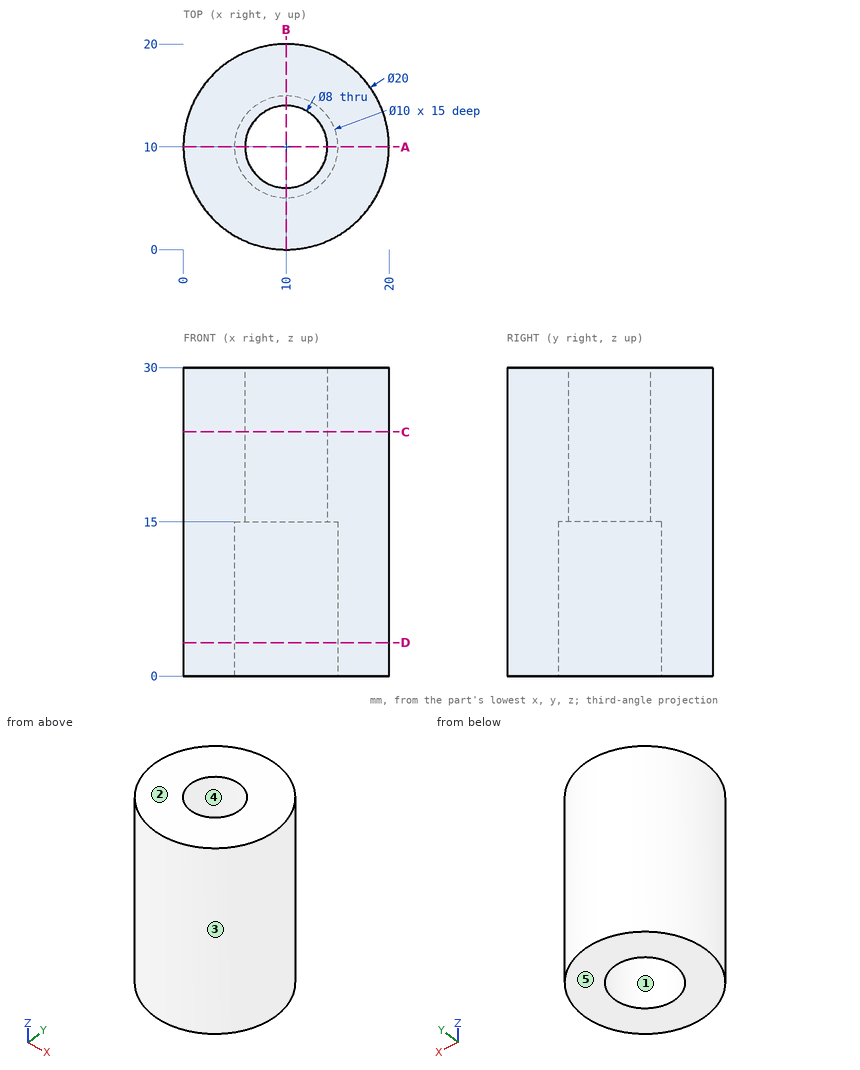
Can you work these out from the drawing? Everything is in mm from the part's minimum corner. A direction names the side the tool comes from. Round coordinates to 2 decimals unless told otherwise and drop trailing zeros. Loops run counter-clockwise (first coordinate to the right, second up) from the corner with the lowest first, then second, coordinate; pieces in that order, holes last. Notation, with made-up numbers: M 38.5,1 L 81.5,1 A13 cw 81.5,22 Z; hole C -36,77.5 d10. An arc over 180 degrees is marked long. Answer in a Markdown table with one row per item.
1. Please list where these lines run through material, in increasing order: line 1 (Y direction, x = 10, z = 11.5); line 2 (Y direction, x = 10, z = 20.5); line 3 (X direction, y = 12.25, z = 27.5). Write a range as from..to.
Established:
| item | result |
|---|---|
| line 1 | 0..5, 15..20 |
| line 2 | 0..6, 14..20 |
| line 3 | 0.26..6.69, 13.31..19.74 |
2. If we section it at C-C, the plane z = 23.75: Please give me the cut outline in (x, y).
Established:
| item | result |
|---|---|
| outline | C 10,10 d20; hole C 10,10 d8 |
3. If we section it at D-D, the plane z = 3.25: Please give me the cut outline in (x, y), plus the area to 3 significant figures.
Established:
| item | result |
|---|---|
| outline | C 10,10 d20; hole C 10,10 d10 |
| area | 236 mm² |
4. On a 3-axis mill with a long thin cutter (end or side, diameter ignored), from which of +Z, -Z, +X, -X, +Y, -Y can I reach the whole of each face in a straight line? I mean the marked faces 1 and 2. Say none if no direction works.
Established:
| item | result |
|---|---|
| face 1 | -Z |
| face 2 | +Z, +X, -X, +Y, -Y |
5. I'm going to push flat-ended pins straight in: pin 1 Ø4 at (y, z) = (14.5, 21) entering from +X; pin 2 Ø1.5 at (x, z) = (12.5, 23.5) entering from +Y; pin 3 Ø11 at (x, y) = (10.5, 11.5) entering from -Z; pin 4 Ø5 at (x, y) = (10, 10) entering from -Z. Where does each tip first touch, or does it pass through?
Established:
| item | result |
|---|---|
| pin 1 | x = 19.68 |
| pin 2 | y = 19.85 |
| pin 3 | z = 0 |
| pin 4 | through |
6. Thinking about a two-plate mould opening in X: for the marked faces 3, 4 and 5, which applies, pulls with the +X half, pulls with the -X half, needs draft (parallel to the pull), parting line crosses it, or undercut?
Established:
| item | result |
|---|---|
| face 3 | parting line crosses it |
| face 4 | undercut |
| face 5 | needs draft |
7. If we section it at A-A, the plane y = 10: Please give me the cut outline in (x, z).
Established:
| item | result |
|---|---|
| outline | M 0,0 L 5,0 L 5,15 L 6,15 L 6,30 L 0,30 Z; M 14,15 L 15,15 L 15,0 L 20,0 L 20,30 L 14,30 Z |
